Can you work these out from the model? Positions are in its coordinate system, mm. Face numbers are marked on the shaded views. Round coordinates to 2 decimals unless told otherwise and drop trailing zeros. Loops run counter-clockwise (first coordinate to the right, second up) from the corner with the lowest first, then second, coordinate; pieces in that order, holes last. Notation, with made-up numbers: (29.5, -20) -> (81.5, -20) arc R17 cw to (81.5, 11) -> close; hole circle Ø11 at (-35.5, 89.5). An arc over 180 degrees is marked (long way). Write item = value, one per line.
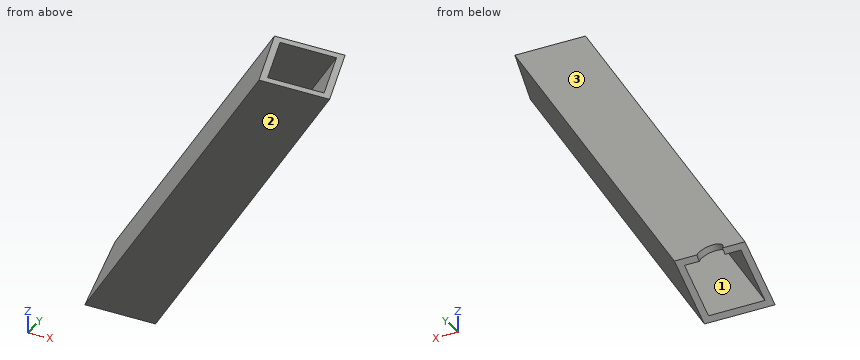
from build123d import *

# Parameters (mm, degrees)
F4_W      = 30
F4_H      = 30
F4_W_2    = 24
F4_H_2    = 24
F5_DEPTH  = 1000
F7_W      = 1359.9022671681
F7_H      = 1462.2605508027
F8_DEPTH  = 477.3996029769
F11_W     = 260.7968747616
F11_H     = 228.6183834076
F12_DEPTH = 46.9924863148
F13_R     = 6.3105959623
F14_DEPTH = 3


with BuildPart() as f5:
    # F4 (on face) → F5 (new body)
    with BuildSketch(Plane(origin=(0, 0, 0), x_dir=(0.8660254038, 0.2753467822, -0.4173537463), z_dir=(0.5, -0.4769146164, 0.7228778933))):
        Rectangle(F4_W, F4_H)
        Rectangle(F4_W_2, F4_H_2, mode=Mode.SUBTRACT)
    extrude(amount=F5_DEPTH)

    # F7 (on offset) → F8 (cut, through all)
    with BuildSketch(Plane.XY.offset(260)):
        with Locations((509.8009683141, -255.676958236)):
            Rectangle(F7_W, F7_H)
    extrude(amount=F8_DEPTH, mode=Mode.SUBTRACT)

    # F11 (on face) → F12 (cut, through all)
    with BuildSketch(Plane(origin=(0, -17.1818181667, 18.1599869076), x_dir=(1, 0, 0), z_dir=(0, -0.6872727267, 0.7263994763))):
        Rectangle(F11_W, F11_H)
    extrude(amount=-F12_DEPTH, mode=Mode.SUBTRACT)

    # F13 (on face) → F14 (cut, through all)
    with BuildSketch(Plane(origin=(0, 12.5206123889, 8.2604034651), x_dir=(-1, 0, 0), z_dir=(0, 0.8347074926, 0.5506935643))):
        with Locations((-16.1834571395, 28.0305700078)):
            Circle(F13_R)
    extrude(amount=-F14_DEPTH, mode=Mode.SUBTRACT)


solid = f5.part
1. Suppose I cut it at A-A, the plane x = 39. List the corners of the cut face in (y, z) for me, and give its area (3 significant figures).
Entries:
outline = (-66.24, 73.17) -> (-33.2, 23.08) -> (-8.16, 39.6) -> (-41.2, 89.69) -> close; hole (-60.43, 69.81) -> (-34, 29.74) -> (-13.97, 42.96) -> (-40.4, 83.03) -> close
area = 648 mm²
2. Suppose I cut it at C-C, the plane x = 185. List the corners of the cut face in (y, z) for me, and give its area (3 significant figures).
Entries:
outline = (-189.5, 260) -> (-172.46, 234.16) -> (-147.42, 250.68) -> (-153.56, 260) -> (-157.16, 260) -> (-153.23, 254.04) -> (-173.26, 240.82) -> (-185.91, 260) -> close
area = 270 mm²
3. I need wall thicknesses on line 1 (Y direction, x = 180.5, z = 248.5); line 2 (Z direction, x = 29, y = -36.5); line 3 (Z direction, x = 112, y = -103.5). Which ranges of each line are inside material? Lowest first, please. Write a range as [from, to].
Entries:
line_1 = [-181.92, -178.32], [-149.57, -145.98]
line_2 = [28.09, 33.53], [64.85, 72.04]
line_3 = [129.64, 135.37], [178.67, 184.12]
4. We'd pull the mould along Z, two halves only. Please class the marked faces 1, 2 and 3: released by +Z, released by -Z, zero draft, split by the parting line, or undercut.
Entries:
face_1 = undercut
face_2 = released by -Z
face_3 = released by +Z
5. Suppose I cut it at B-B, the plane y = -77. List the corners of the cut face in (x, z) for me (1 decimal), and give its area (3 significant figures).
Entries:
outline = (50.3, 89.5) -> (84.9, 89.5) -> (111.2, 144) -> (76.5, 144) -> close; hole (56.4, 94.9) -> (84.1, 94.9) -> (105.1, 138.5) -> (77.4, 138.5) -> close
area = 679 mm²
6. I'm going to push flat-ended pins straight in: pin 1 (12 mm diameter, centred on x = 163.5, y = -139.5, fed in from -Z); pin 2 (3 mm diameter, centred on x = 128, y = -100.5, fed in from -Z); pin 3 (2 mm diameter, centred on x = 48.5, z = 51.5, fed in from -Y). Where does each tip first touch, or does it pass through?
Entries:
pin_1 = 198.23
pin_2 = 160.09
pin_3 = -52.61
